Geometry check sheet. Reference: the model listing, model coordinates, mm. Face numbers are marked on the shaded views. A direction names the side the tool comes from. Give positions to 0.01 mm unless a question says otherwise; leave off trailing zeros. Order: outer loops, then holes, each group sorted by start corner. A loop starts at its lowest first (then second) coordinate and runs counter-clockwise, first axis right, second up. Notation, with made-up numbers: M 13.5,18 L 35.5,18 A25 cw 35.5,53 Z; hole C -11,41 d7. An arc over 180 degrees is marked long. One line per question, with ' | ' between items. Start each with the question number.
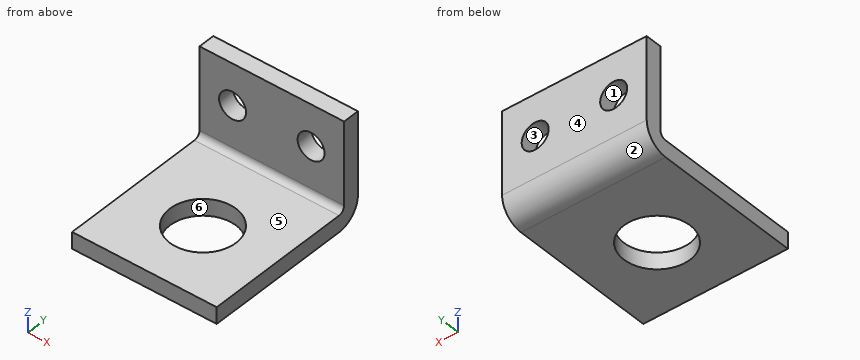
from build123d import *

# Parameters (mm, degrees)
SKETCH1_W                 = 17.5
SKETCH1_H                 = 10
BASE_FLANGE1_DEPTH        = 2
F_4_CLEARANCE_HOLE1_D     = 3.2639
F_4_CLEARANCE_HOLE1_DEPTH = 2
F_4_CLEARANCE_HOLE1_TIP   = 0.980574487
EDGE_FLANGE1_DEPTH        = 17.5
SKETCH20_R                = 4
CUT_EXTRUDE1_DEPTH        = 2


# Sheet-metal steps are written as plain solids
with BuildPart() as part:
    # Sketch1 → Base-Flange1 (new body)
    with BuildSketch(Plane(origin=(0, 0, 0), x_dir=(1, 0, 0), z_dir=(0, 1, 0))):
        with Locations((-14.536713287, 16.32983683)):
            Rectangle(SKETCH1_W, SKETCH1_H)
    extrude(amount=-BASE_FLANGE1_DEPTH)

    # #4 Clearance Hole1
    with Locations(Plane.XZ.offset(2)):
        with Locations((-9.786713287, -16.32983683), (-19.286713287, -16.32983683)):
            Hole(F_4_CLEARANCE_HOLE1_D / 2, depth=F_4_CLEARANCE_HOLE1_DEPTH)
            with Locations((0, 0, -(F_4_CLEARANCE_HOLE1_DEPTH + F_4_CLEARANCE_HOLE1_TIP / 2))):  # 118° drill point
                Cone(0, F_4_CLEARANCE_HOLE1_D / 2, F_4_CLEARANCE_HOLE1_TIP, mode=Mode.SUBTRACT)

    # Edge-Flange1 section (across the edge) → Edge-Flange1 (add)
    with BuildSketch(Plane(origin=(-23.286713287, -2, -22.06643683), x_dir=(0, 0, 1), z_dir=(1, 0, 0))):
        with BuildLine():
            Line((-2, 0.7366), (-2, 18.5))
            Line((-2, 18.5), (0, 18.5))
            Line((0, 18.5), (0, 0.7366))
            ThreePointArc((0, 0.7366), (0.215745145, 0.215745145), (0.7366, 0))
            Line((0.7366, 0), (0.7366, -2))
            ThreePointArc((0.7366, -2), (-1.198468417, -1.198468417), (-2, 0.7366))
        make_face()
    extrude(amount=EDGE_FLANGE1_DEPTH)

    # Sketch20 → Cut-Extrude1 (cut)
    with BuildSketch(Plane(origin=(0, 0, -24.06643683), x_dir=(-1, 0, 0), z_dir=(0, 0, -1))):
        with Locations(Location((14.536713287, -12, 0), (0, 0, 90))):
            Circle(SKETCH20_R)
    extrude(amount=-CUT_EXTRUDE1_DEPTH, mode=Mode.SUBTRACT)


solid = part.part
Item 1: Mould release check, pull along Z, two halves, no side actions. Record for the marked faces 1, 2, 3 and 4: released by +Z, released by -Z, zero draft, split by the parting line, or undercut.
Item 2: Material ranges on line 1 along X through (y, z) = (-12, -22.9); line 2 along Z through (x, y) = (-9.5, -12.75); line 3 along Y through (x, z) = (-6.5, -18), recorded low to high.
Item 3: Depth check by flat-ended pin: pin 1 (9 mm diameter, centred on x = -10.5, y = -12, fed in from +Z); pin 2 (4 mm diameter, centred on x = -9.79, z = -16.33, fed in from -Y). Enter the tip coordinate at first touch or a pass-through.
Item 4: Set-up check for the marked faces 5 and 6: record each of +Z, -Z, +X, -X, +Y, -Y from which the full face is reachable in a straight line by a thin tool's end or side.
Item 5: Cross-section at A-A, the plane y = -9.75. Record the cut outline in (x, z).
Item 6: Cross-section at D-D, the plane y = -12. Record the cut outline in (x, z).
Item 7: Cross-section at B-B, the plane z = -17. Record the cut outline in (x, y), plus the area to 3 significant figures.
Item 8: Cross-section at C-C, the plane x = -18.25. Record the cut outline in (y, z), plus the area to 3 significant figures.
Outcome:
1) face 1: undercut | face 2: released by -Z | face 3: undercut | face 4: zero draft
2) line 1: x = -23.29 to -18.54, -10.54 to -5.79 | line 2: z = -24.07 to -22.07 | line 3: y = -2 to 0
3) pin 1: stops at z = -22.07 | pin 2: stops at y = -2
4) face 5: +Z, +X, -X, -Y | face 6: +Z, -Z
5) outline: M -23.29,-24.07 L -17.84,-24.07 L -17.84,-22.07 L -23.29,-22.07 Z; M -11.23,-24.07 L -5.79,-24.07 L -5.79,-22.07 L -11.23,-22.07 Z
6) outline: M -23.29,-24.07 L -18.54,-24.07 L -18.54,-22.07 L -23.29,-22.07 Z; M -10.54,-24.07 L -5.79,-24.07 L -5.79,-22.07 L -10.54,-22.07 Z
7) outline: M -23.29,-2 L -20.77,-2 L -20.77,0 L -23.29,0 Z; M -17.8,-2 L -11.27,-2 L -11.27,0 L -17.8,0 Z; M -8.3,-2 L -5.79,-2 L -5.79,0 L -8.3,0 Z | area: 23.1 mm²
8) outline: M -20.5,-24.07 L -13.49,-24.07 L -13.49,-22.07 L -20.5,-22.07 Z; M -10.51,-24.07 L -2.74,-24.07 A2.74 ccw 0,-21.33 L 0,-17.59 L -2,-17.59 L -2,-21.33 A0.74 cw -2.74,-22.07 L -10.51,-22.07 Z; M -2,-15.07 L 0,-15.07 L 0,-11.33 L -2,-11.33 Z | area: 50.0 mm²
